The listing builds one solid part. Answer for the finished solid, in the listing's coordinates (mm). A direction names the side the tool comes from. Give positions to 0.01 mm unless a question says otherwise; leave off trailing zeros. Write each loop counter-clockwise with the first axis right and the second up, starting at its lowest first coordinate (ties: lowest second). Pieces come first, ordered by that corner, then holes.
```python
from build123d import *

# Parameters (mm, degrees)
ESQUISSE1_W                = 85
ESQUISSE1_H                = 56
BOSS_EXTRU_1_DEPTH         = 1
CONG_3_R                   = 3
CONG_4_R                   = 3
CONG_5_R                   = 3
CONG_6_R                   = 3
ESQUISSE2_R                = 1.5
ENL_V_MAT_EXTRU_1_DEPTH    = 55.498557908
ESQUISSE3_W                = 15.3
ESQUISSE3_H                = 13.6
BOSS_EXTRU_3_DEPTH         = 16
ESQUISSE5_W                = 16
ESQUISSE5_H                = 13.6
BOSS_EXTRU_4_DEPTH         = 2.7
R_P_TITION_LIN_AIRE1_COUNT = 2
R_P_TITION_LIN_AIRE1_PITCH = 18
R_P_TITION_LIN_AIRE2_COUNT = 2
R_P_TITION_LIN_AIRE2_PITCH = 18
ESQUISSE7_W                = 21.7
ESQUISSE7_H                = 15.4
BOSS_EXTRU_5_DEPTH         = 13.5
ESQUISSE8_W                = 6.8
ESQUISSE8_H                = 15
BOSS_EXTRU_6_DEPTH         = 6
ESQUISSE9_W                = 14.5
ESQUISSE9_H                = 16.7
BOSS_EXTRU_7_DEPTH         = 6.5
ESQUISSE10_W               = 8.15
ESQUISSE10_H               = 5.88
BOSS_EXTRU_8_DEPTH         = 1.8


with BuildPart() as part:
    # Esquisse1 → Boss.-Extru.1 (new body)
    with BuildSketch(Plane.XY):
        with Locations((-1.608108108, -3.993243243)):
            Rectangle(ESQUISSE1_W, ESQUISSE1_H)
    extrude(amount=BOSS_EXTRU_1_DEPTH)

    # Congé3
    cong_3_edges = [part.edges().sort_by_distance(p)[0] for p in [
        (40.891891892, 24.006756757, 0.5),
    ]]
    fillet(cong_3_edges, radius=CONG_3_R)

    # Congé4
    cong_4_edges = [part.edges().sort_by_distance(p)[0] for p in [
        (-44.108108108, 24.006756757, 0.5),
    ]]
    fillet(cong_4_edges, radius=CONG_4_R)

    # Congé5
    cong_5_edges = [part.edges().sort_by_distance(p)[0] for p in [
        (-44.108108108, -31.993243243, 0.5),
    ]]
    fillet(cong_5_edges, radius=CONG_5_R)

    # Congé6
    cong_6_edges = [part.edges().sort_by_distance(p)[0] for p in [
        (40.891891892, -31.993243243, 0.5),
    ]]
    fillet(cong_6_edges, radius=CONG_6_R)

    # Esquisse2 → Enlèv. mat.-Extru.1 (cut, through all)
    with BuildSketch(Plane.XY.offset(1)):
        with Locations((-40.608108108, 20.506756757)):
            Circle(ESQUISSE2_R)
        with Locations((-40.608108108, -28.493243243)):
            Circle(ESQUISSE2_R)
        with Locations((17.391891892, -28.493243243)):
            Circle(ESQUISSE2_R)
        with Locations((17.391891892, 20.506756757)):
            Circle(ESQUISSE2_R)
    extrude(amount=-ENL_V_MAT_EXTRU_1_DEPTH, mode=Mode.SUBTRACT)

    # Esquisse3 → Boss.-Extru.3 (add)
    with BuildSketch(Plane.XY.offset(1)):
        with Locations((33.241891892, 15.006756757)):
            Rectangle(ESQUISSE3_W, ESQUISSE3_H)
    boss_extru_3 = extrude(amount=BOSS_EXTRU_3_DEPTH)

    # Esquisse5 → Boss.-Extru.4 (add)
    with BuildSketch(Plane(origin=(40.891891892, 0, 0), x_dir=(0, 0, -1), z_dir=(1, 0, 0))):
        with Locations((-9, 15.006756757)):
            Rectangle(ESQUISSE5_W, ESQUISSE5_H)
    boss_extru_4 = extrude(amount=BOSS_EXTRU_4_DEPTH)

    # Répétition linéaire1: Boss.-Extru.3 ×2
    with Locations(*[(0, -i * R_P_TITION_LIN_AIRE1_PITCH, 0) for i in range(1, R_P_TITION_LIN_AIRE1_COUNT)]):
        add(boss_extru_3)

    # Répétition linéaire2: Boss.-Extru.4 ×2
    with Locations(*[(0, -i * R_P_TITION_LIN_AIRE2_PITCH, 0) for i in range(1, R_P_TITION_LIN_AIRE2_COUNT)]):
        add(boss_extru_4)

    # Esquisse7 → Boss.-Extru.5 (add)
    with BuildSketch(Plane.XY.offset(1)):
        with Locations((32.741891892, -21.743243243)):
            Rectangle(ESQUISSE7_W, ESQUISSE7_H)
    extrude(amount=BOSS_EXTRU_5_DEPTH)

    # Esquisse8 → Boss.-Extru.6 (add)
    with BuildSketch(Plane.XY.offset(1)):
        with Locations((9.391891892, -27.693243243)):
            Rectangle(ESQUISSE8_W, ESQUISSE8_H)
    extrude(amount=BOSS_EXTRU_6_DEPTH)

    # Esquisse9 → Boss.-Extru.7 (add)
    with BuildSketch(Plane.XY.offset(1)):
        with Locations((-10.491721189, -25.443243243)):
            Rectangle(ESQUISSE9_W, ESQUISSE9_H)
    extrude(amount=BOSS_EXTRU_7_DEPTH)

    # Esquisse10 → Boss.-Extru.8 (add)
    with BuildSketch(Plane.XY.offset(1)):
        with Locations((-29.658093883, -30.413243243)):
            Rectangle(ESQUISSE10_W, ESQUISSE10_H)
    extrude(amount=BOSS_EXTRU_8_DEPTH)


solid = part.part
```
Item 1: A cutting plane is placed at D-D, the plane y = -22. Give the vertices of the cut face in (x, z), plus the area to 3 significant figures.
Conclusion:
outline: (-44.11, 0) - (40.89, 0) - (40.89, 1) - (43.59, 1) - (43.59, 14.5) - (21.89, 14.5) - (21.89, 1) - (12.79, 1) - (12.79, 7) - (5.99, 7) - (5.99, 1) - (-3.24, 1) - (-3.24, 7.5) - (-17.74, 7.5) - (-17.74, 1) - (-44.11, 1) - close
area: 513 mm2
Item 2: A cutting plane is placed at C-C, the plane z = 3.75. Give the vertices of the cut face in (x, y).
Conclusion:
outline: (-17.74, -33.79) - (-3.24, -33.79) - (-3.24, -17.09) - (-17.74, -17.09) - close; (5.99, -35.19) - (12.79, -35.19) - (12.79, -20.19) - (5.99, -20.19) - close; (21.89, -29.44) - (43.59, -29.44) - (43.59, -14.04) - (21.89, -14.04) - close; (25.59, -9.79) - (43.59, -9.79) - (43.59, 3.81) - (25.59, 3.81) - close; (25.59, 8.21) - (43.59, 8.21) - (43.59, 21.81) - (25.59, 21.81) - close
Item 3: Consider probe 1 along Y at (x, z) = (26, 9); probe 2 along X at (y, z) = (-23.5, 6.5); probe 3 along X at (y, z) = (-18.5, 1.5). Determine where each line is inside the solid, lowest interval first.
Conclusion:
probe 1: y = -29.44 to -14.04, -9.79 to 3.81, 8.21 to 21.81
probe 2: x = -17.74 to -3.24, 5.99 to 12.79, 21.89 to 43.59
probe 3: x = -17.74 to -3.24, 21.89 to 43.59
Item 4: Which of the six approach directions +Z, -Z, +X, -X, +Y, -Y give full straight-line access (tool end or side, diameter ignored) to faces 1 (the face through (9, -34, 1)), 2 (the face through (-11, -25, 7.5)), 3 (the face through (42, -22, 1)), 4 (the face through (33, -14.043, 8))?
Conclusion:
face 1: -Z, +X, -X, -Y
face 2: +Z, -X, +Y, -Y
face 3: -Z, +X, +Y, -Y
face 4: +Z, +X, -X
Item 5: A cutting plane is placed at B-B, the plane x = -13. Give the vertices of the cut face in (y, z).
Conclusion:
outline: (-33.79, 1) - (-31.99, 1) - (-31.99, 0) - (24.01, 0) - (24.01, 1) - (-17.09, 1) - (-17.09, 7.5) - (-33.79, 7.5) - close
Item 6: Each of these flat-tipped pins is pushed along its axis until it touches: P1, Ø1.5, axis at x = 14.5, y = -2, coming from the -Z side; P2, Ø2, axis at x = 21, z = 8, coming from the -Y side; P3, Ø0.8, axis at y = 4.5, z = 0.5, coming from the +X side; P4, Ø0.9, axis at y = -31, z = 1.5, coming from the -X side. Where does it stop, or does it pass through?
Conclusion:
P1: stops at z = 0
P2: stops at y = -29.44
P3: stops at x = 40.89
P4: stops at x = -33.73
Item 7: A cutting plane is placed at A-A, the plane z = 11.25. Give the vertices of the cut face in (x, y).
Conclusion:
outline: (21.89, -29.44) - (43.59, -29.44) - (43.59, -14.04) - (21.89, -14.04) - close; (25.59, -9.79) - (43.59, -9.79) - (43.59, 3.81) - (25.59, 3.81) - close; (25.59, 8.21) - (43.59, 8.21) - (43.59, 21.81) - (25.59, 21.81) - close
Item 8: Determine the mould class of faces 5 (the face through (43.592, -3, 9)), 6 (the face through (34, -3, 17)), 7 (the face through (-3.242, -26, 4)) for opening direction X: pulls with the +X half, pulls with the -X half, needs draft (parallel to the pull), parting line crosses it, or undercut.
Conclusion:
face 5: pulls with the +X half
face 6: needs draft
face 7: undercut
